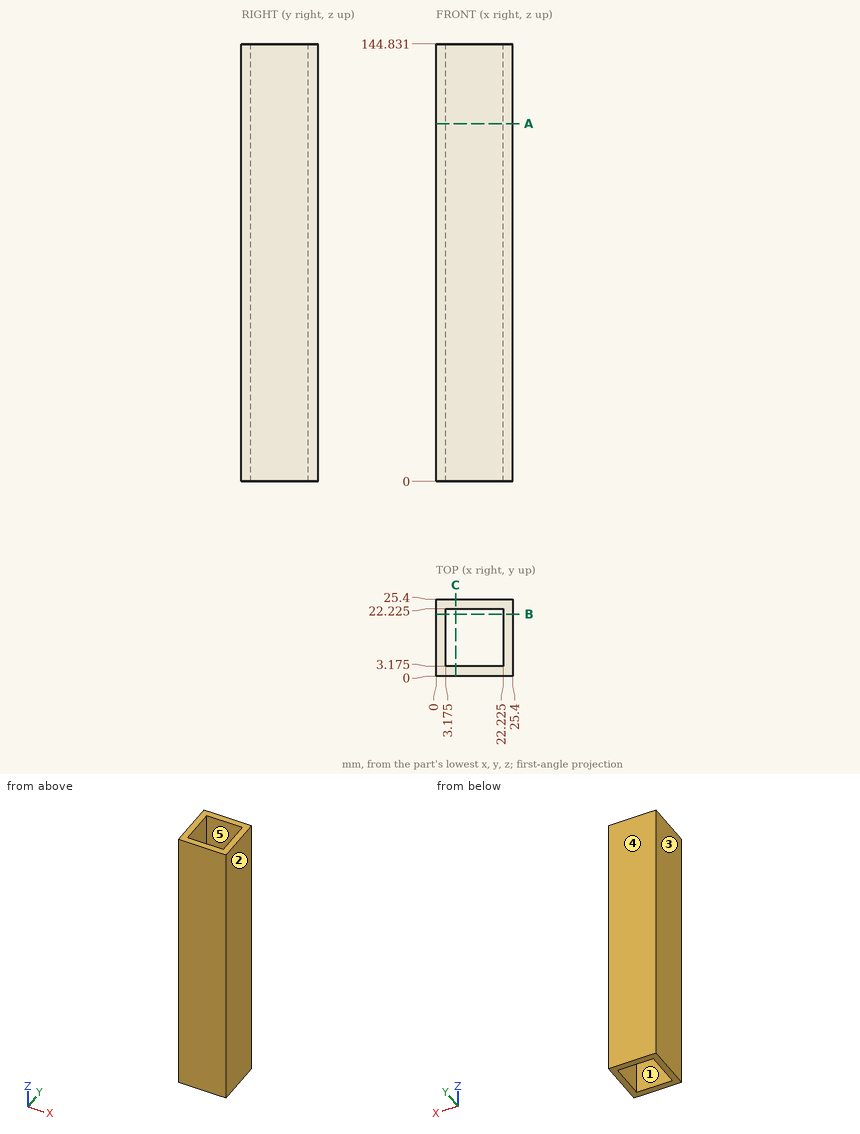
Check sheet for the drawn part. Datum: minimum x, y, z corner. Units: mm. A direction names the side the tool comes from. Round coordinates to 2 decimals unless told otherwise and drop trailing zeros. Loops run counter-clockwise (first coordinate to the right, second up) from the corner with the lowest first, then second, coordinate; pieces in that order, holes last. Notation, with made-up numbers: (-18.75, 6.25) - (5.25, 6.25) arc R24 ccw to (5.25, 29.25) - close; hole circle Ø8 at (7, -38). An arc over 180 degrees is marked (long way). Write each question's results on one line, items separated by ' | '. Start each with the question number.
Q1. Release check for a two-part mould opening along Y. For the marked faces 3, 4 and 5 record: +Y half, -Y half, draft (parallel to the pull), parting line (faces both ways), or undercut.
Q2. Access from +Z, -Z, +X, -X, +Y, -Y to the whole of each face (thin tool, end or side, straight path). Record for the marked faces 1 and 2.
Q3. Cross-section at A-A on z = 118.5. Enter the section's corners in (x, y) (3 decimals).
Q4. Cross-section at B-B on y = 20.5. Enter the section's corners in (x, z) (1 decimal).
Q5. Thickness scan on line 1 (X direction, y = 22, z = 86.5) (3 decimals). Record the ranges inside material, lowest first. Write a range as [from, to].
Answers below:
1) face 3: draft | face 4: +Y half | face 5: undercut
2) face 1: +Z, -Z | face 2: +Z, -Z, +X, +Y, -Y
3) outline: (0, 0) - (25.4, 0) - (25.4, 25.4) - (0, 25.4) - close; hole (3.175, 3.175) - (22.225, 3.175) - (22.225, 22.225) - (3.175, 22.225) - close
4) outline: (0, 0) - (3.2, 0) - (3.2, 144.8) - (0, 144.8) - close; (22.2, 0) - (25.4, 0) - (25.4, 144.8) - (22.2, 144.8) - close
5) line 1: x = [0, 3.175], [22.225, 25.4]
